```python
from build123d import *

# Parameters (mm, degrees)
F1_DEPTH = 4.9
F2_D     = 3.5


with BuildPart() as f1:
    # F0 (on Top) → F1 (new body)
    with BuildSketch(Plane.XY):
        with BuildLine():
            ThreePointArc((-2.4513349141, 5.8753238716), (-2.436238396, 5.8815997768), (-2.4211258105, 5.887836892))
            ThreePointArc((-2.4211258105, 5.887836892), (-6.2693485338, 6.2693485338), (-5.887836892, 2.4211258105))
            ThreePointArc((-5.887836892, 2.4211258105), (-5.8815997768, 2.436238396), (-5.8753238716, 2.4513349141))
            ThreePointArc((-5.8753238716, 2.4513349141), (-5.2887540631, 3.5436639114), (-4.5015815808, 4.5015815808))
            ThreePointArc((-4.5015815808, 4.5015815808), (-3.5436639114, 5.2887540631), (-2.4513349141, 5.8753238716))
        make_face()
        with BuildLine():
            ThreePointArc((2.4513349141, 5.8753238716), (4.5015815808, 4.5015815808), (5.8753238716, 2.4513349141))
            ThreePointArc((5.8753238716, 2.4513349141), (5.8815997768, 2.436238396), (5.887836892, 2.4211258105))
            ThreePointArc((5.887836892, 2.4211258105), (6.7056276645, 3.32167444), (7.0015815808, 4.5015815808))
            ThreePointArc((7.0015815808, 4.5015815808), (5.2257571722, 6.8943978531), (2.4211258105, 5.887836892))
            ThreePointArc((2.4211258105, 5.887836892), (2.436238396, 5.8815997768), (2.4513349141, 5.8753238716))
        make_face()
        with BuildLine():
            ThreePointArc((4.9155755495, -2.0360980595), (3.8661977237, 0), (4.9155755495, 2.0360980595))
            ThreePointArc((4.9155755495, 2.0360980595), (2.7338146278, 2.7338146278), (2.0360980595, 4.9155755495))
            ThreePointArc((2.0360980595, 4.9155755495), (0, 3.8661977237), (-2.0360980595, 4.9155755495))
            ThreePointArc((-2.0360980595, 4.9155755495), (-2.0102256444, 4.7092967665), (-2.0015815808, 4.5015815808))
            ThreePointArc((-2.0015815808, 4.5015815808), (-2.1918827495, 3.5448729999), (-2.7338146278, 2.7338146278))
            ThreePointArc((-2.7338146278, 2.7338146278), (-3.7400847484, 2.1203796628), (-4.9155755495, 2.0360980595))
            ThreePointArc((-4.9155755495, 2.0360980595), (-3.8661977237, 0), (-4.9155755495, -2.0360980595))
            ThreePointArc((-4.9155755495, -2.0360980595), (-2.8868037202, -2.5930500875), (-2.0015815808, -4.5015815808))
            ThreePointArc((-2.0015815808, -4.5015815808), (-2.0102256444, -4.7092967665), (-2.0360980595, -4.9155755495))
            ThreePointArc((-2.0360980595, -4.9155755495), (0, -3.8661977237), (2.0360980595, -4.9155755495))
            ThreePointArc((2.0360980595, -4.9155755495), (2.7338146278, -2.7338146278), (4.9155755495, -2.0360980595))
        make_face()
        with BuildLine():
            ThreePointArc((7.0015815808, -4.5015815808), (6.7056276645, -3.32167444), (5.887836892, -2.4211258105))
            ThreePointArc((5.887836892, -2.4211258105), (5.8815997768, -2.436238396), (5.8753238716, -2.4513349141))
            ThreePointArc((5.8753238716, -2.4513349141), (4.5015815808, -4.5015815808), (2.4513349141, -5.8753238716))
            ThreePointArc((2.4513349141, -5.8753238716), (2.436238396, -5.8815997768), (2.4211258105, -5.887836892))
            ThreePointArc((2.4211258105, -5.887836892), (5.2257571722, -6.8943978531), (7.0015815808, -4.5015815808))
        make_face()
        with BuildLine():
            ThreePointArc((-5.8753238716, -2.4513349141), (-5.8815997768, -2.436238396), (-5.887836892, -2.4211258105))
            ThreePointArc((-5.887836892, -2.4211258105), (-6.2693485338, -6.2693485338), (-2.4211258105, -5.887836892))
            ThreePointArc((-2.4211258105, -5.887836892), (-2.436238396, -5.8815997768), (-2.4513349141, -5.8753238716))
            ThreePointArc((-2.4513349141, -5.8753238716), (-4.5015815808, -4.5015815808), (-5.8753238716, -2.4513349141))
        make_face()
        with BuildLine():
            ThreePointArc((4.9155755495, 2.0360980595), (5.3734957964, 2.2944591702), (5.8753238716, 2.4513349141))
            ThreePointArc((5.8753238716, 2.4513349141), (4.5015815808, 4.5015815808), (2.4513349141, 5.8753238716))
            ThreePointArc((2.4513349141, 5.8753238716), (2.2944591702, 5.3734957964), (2.0360980595, 4.9155755495))
            ThreePointArc((2.0360980595, 4.9155755495), (2.7338146278, 2.7338146278), (4.9155755495, 2.0360980595))
        make_face()
        with BuildLine():
            Line((-2.7338146278, 2.7338146278), (-4.5015815808, 4.5015815808))
            ThreePointArc((-4.5015815808, 4.5015815808), (-5.2887540631, 3.5436639114), (-5.8753238716, 2.4513349141))
            ThreePointArc((-5.8753238716, 2.4513349141), (-5.3734957964, 2.2944591702), (-4.9155755495, 2.0360980595))
            ThreePointArc((-4.9155755495, 2.0360980595), (-3.7400847484, 2.1203796628), (-2.7338146278, 2.7338146278))
        make_face()
        with BuildLine():
            ThreePointArc((-2.4513349141, -5.8753238716), (-2.2944591702, -5.3734957964), (-2.0360980595, -4.9155755495))
            ThreePointArc((-2.0360980595, -4.9155755495), (-2.0102256444, -4.7092967665), (-2.0015815808, -4.5015815808))
            ThreePointArc((-2.0015815808, -4.5015815808), (-2.8868037202, -2.5930500875), (-4.9155755495, -2.0360980595))
            ThreePointArc((-4.9155755495, -2.0360980595), (-5.3734957964, -2.2944591702), (-5.8753238716, -2.4513349141))
            ThreePointArc((-5.8753238716, -2.4513349141), (-4.5015815808, -4.5015815808), (-2.4513349141, -5.8753238716))
        make_face()
        with BuildLine():
            ThreePointArc((-2.0015815808, 4.5015815808), (-2.0102256444, 4.7092967665), (-2.0360980595, 4.9155755495))
            ThreePointArc((-2.0360980595, 4.9155755495), (-2.2944591702, 5.3734957964), (-2.4513349141, 5.8753238716))
            ThreePointArc((-2.4513349141, 5.8753238716), (-3.5436639114, 5.2887540631), (-4.5015815808, 4.5015815808))
            Line((-4.5015815808, 4.5015815808), (-2.7338146278, 2.7338146278))
            ThreePointArc((-2.7338146278, 2.7338146278), (-2.1918827495, 3.5448729999), (-2.0015815808, 4.5015815808))
        make_face()
        with BuildLine():
            ThreePointArc((5.8753238716, -2.4513349141), (5.3734957964, -2.2944591702), (4.9155755495, -2.0360980595))
            ThreePointArc((4.9155755495, -2.0360980595), (2.7338146278, -2.7338146278), (2.0360980595, -4.9155755495))
            ThreePointArc((2.0360980595, -4.9155755495), (2.2944591702, -5.3734957964), (2.4513349141, -5.8753238716))
            ThreePointArc((2.4513349141, -5.8753238716), (4.5015815808, -4.5015815808), (5.8753238716, -2.4513349141))
        make_face()
    extrude(amount=F1_DEPTH)

    # F2 (through all)
    with Locations(Plane(origin=(0, 0, 0), x_dir=(1, 0, 0), z_dir=(0, 0, -1))):
        with Locations((0, 0)):
            Hole(F2_D / 2)


solid = f1.part
```
Can you work these out from the model? Positions are in its coordinate system, mm. Round coordinates to 2 decimals unless told otherwise and drop trailing zeros. Order: outer loops, then holes, each group sorted by start corner. A loop starts at its lowest first (then second) coordinate and runs counter-clockwise, first axis right, second up. Notation, with made-up numbers: (6, 49) -> (24, 49) arc R33 ccw to (24, 84) -> close; hole circle Ø4 at (79, 4). An arc over 180 degrees is marked (long way). Return JSON: item names as keys, results as strings. Group by question number.
1. If we section it at D-D, the plane x = 2.25: Write out the boundary of the cut face in (y, z), then the cut area to 3 significant figures.
2. We'd pull the mould along X, two halves only. Please class faces 1 (the face through (-1.617, 0.67, 2.484)), 2 (the face through (-6.23, 6.31, 2.42)), 3 (the face through (1.5, -1.5, 4.9)): released by +X, released by -X, zero draft, split by the parting line, or undercut.
3. Will this pin go through, and if not, where does the flat tip stop? pin 1 (1 mm diameter, centred on y = 1, z = 3, fed in from +X).
4. I need wall thicknesses on line 1 (X direction, y = -5.25, z = 3.75); line 2 (Y direction, x = 4.75, z = 2.85); line 3 (X direction, y = 1.5, z = 3.5). Which ranges of each line are inside material? Lowest first, please. Write a range as [from, to].
5. If we section it at A-A, the plane y = 0: Write out the boundary of the cut face in (x, z).
Output values:
{
 "1": {"outline": "(-5.28, 0) -> (5.28, 0) -> (5.28, 4.9) -> (-5.28, 4.9) -> close", "area": "51.7 mm²"},
 "2": {"face 1": "undercut", "face 2": "undercut", "face 3": "zero draft"},
 "3": {"pin 1": "x = 4.37"},
 "4": {"line 1": "[-6.89, -2.24], [2.24, 6.89]", "line 2": "[-6.99, -1.91], [1.91, 6.99]", "line 3": "[-4.37, -0.9], [0.9, 4.37]"},
 "5": {"outline": "(-3.87, 0) -> (-1.75, 0) -> (-1.75, 4.9) -> (-3.87, 4.9) -> close; (1.75, 0) -> (3.87, 0) -> (3.87, 4.9) -> (1.75, 4.9) -> close"}
}
